The listing builds one solid part. Answer for the finished solid, in the listing's coordinates (mm). A direction names the side the tool comes from. Round coordinates to 2 decimals unless told otherwise and drop trailing zeros. Write each loop counter-clockwise with the first axis right and the second up, starting at its lowest first coordinate (ties: lowest second). Pieces come first, ordered by that corner, then holes. Notation, with made-up numbers: M 26,60.5 L 39,60.5 A22 ccw 39,70.5 Z; hole C 49.25,43.25 d1. An arc over 180 degrees is marked long. Write each question's results on one line, items separated by ' | '.
from build123d import *

# Parameters (mm, degrees)
F0_W     = 77.8002
F0_H     = 47.625
F1_DEPTH = 9.525
F3_DEPTH = 9.525


# Not quite as in the source:
# - a pattern or mirror of a feature is missing from the dataset's text; its kind, count and spacing are read off the source's solid


with BuildPart() as f1:
    # F0 (on Top) → F1 (new body)
    with BuildSketch(Plane.XY):
        Rectangle(F0_W, F0_H)
    extrude(amount=F1_DEPTH)

    # F2 (on face) → F3 (join)
    with BuildSketch(Plane.XZ.offset(23.8125)):
        Polygon((-38.9001, 38.1), (-38.9001, 9.525), (38.9001, 9.525), (38.9001, 28.575), (-7.1501, 28.575), (-19.8501, 38.1), align=None)
    f3 = extrude(amount=-F3_DEPTH)

    # F3_copies: F3 across plane
    add(f3.mirror(Plane.ZX))


solid = f1.part
1) Section C-C (y = -21) is taken. Determine the outline of the cut face in (x, z) (3 decimals), then the cut area to 3 significant figures.
Return value:
outline: M -38.9,0 L 38.9,0 L 38.9,28.575 L -7.15,28.575 L -19.85,38.1 L -38.9,38.1 Z | area: 2,470 mm²
2) Find the intervals of material crossed by line 1 (Y direction, x = 19, z = 14.5); line 2 (Z direction, x = 24.5, y = -13) (3 decimals); line 3 (Z direction, x = 14, y = 20.5) (3 decimals), in increasing order.
Return value:
line 1: -23.81 to -14.29, 14.29 to 23.81 | line 2: 0 to 9.525 | line 3: 0 to 28.575
3) This flat-tipped pin is pushed along its axis until it touches: pin 1 (10 mm diameter, centred on x = 29.5, y = 11.5, fed in from +Z) (3 decimals). Where does it stop, or does it pass through?
Return value:
pin 1: z = 28.575
4) The mould has two halves that part along Y. Classify faces 1 (the face through (-1, 14.288, 21)), 2 (the face through (-29, -19, 38.1)), 3 (the face through (-1, -23.812, 15)): +Y half, -Y half, draft (parallel to the pull), parting line (faces both ways), or undercut.
Return value:
face 1: undercut | face 2: draft | face 3: -Y half
5) Section B-B (x = 29.5) is taken. Determine the outline of the cut face in (y, z) (1 decimal).
Return value:
outline: M -23.8,0 L 23.8,0 L 23.8,28.6 L 14.3,28.6 L 14.3,9.5 L -14.3,9.5 L -14.3,28.6 L -23.8,28.6 Z
6) A tool of negligible diameter and unlimited length cuts with its end or side. For faces 4 (the face through (-1, 0, 9.525)), 5 (the face through (16, -19, 28.575)), 6 (the face through (-38.9, 0, 7)), from which of +Z, -Z, +X, -X, +Y, -Y can it reach the whole face along a straight path? Write none if from no direction.
Return value:
face 4: +Z, +X, -X | face 5: +Z, +X, +Y, -Y | face 6: +Z, -Z, -X, +Y, -Y
7) Section A-A (z = 25.5) is taken. Determine the outline of the cut face in (x, y), then the cut area to 3 significant figures.
Return value:
outline: M -38.9,-23.81 L 38.9,-23.81 L 38.9,-14.29 L -38.9,-14.29 Z; M -38.9,14.29 L 38.9,14.29 L 38.9,23.81 L -38.9,23.81 Z | area: 1,480 mm²
8) Section D-D (z = 31) is taken. Determine the outline of the cut face in (x, y).
Return value:
outline: M -38.9,-23.81 L -10.38,-23.81 L -10.38,-14.29 L -38.9,-14.29 Z; M -38.9,14.29 L -10.38,14.29 L -10.38,23.81 L -38.9,23.81 Z
